The model under review builds one solid part; all positions refer to its coordinate system, in mm. A direction names the side the tool comes from. Round coordinates to 2 decimals unless told otherwise and drop trailing zeros. Write each loop counter-clockwise with the first axis right and the second up, starting at its lowest first coordinate (ties: lowest second). Pieces come first, ordered by that corner, then holes.
Item 1: Add section A-A (y = 7). Give the boundary of the cut face in (x, z), plus the area to 3 significant figures.
Item 2: Machinability: for faces 4 (the face through (2, 6, -27)), 5 (the face through (-5.93, 11.055, -13.579)), 6 (the face through (-0.493, 11.562, -13.026)), which of the approach directions +Z, -Z, +X, -X, +Y, -Y give a long, thin tool a straight path to every point of the face, cutting with its end or side? Answer none if there is none.
Item 3: Add section B-B (z = 0). Give the boundary of the cut face in (x, y).
Item 4: Clearance check with flat-ended pins moving along their axes: pin 1 Ø5 at (y, z) = (10, 0) entering from -X; pin 2 Ø3 at (x, y) = (-8.5, 6.5) entering from +Z; pin 3 Ø1.5 at (x, y) = (-6, 4) entering from +Z. State where each tip first meets the part, or that it passes through.
Item 5: Add section C-C (y = 10). Give the boundary of the cut face in (x, z).
Item 6: Add section D-D (x = -3). Give the boundary of the cut face in (y, z).
Item 7: To check wall thickness, follow L1, parallel to Y at x = 1.3, z = 0; L2, parallel to Z at x = 3.05, y = 10; L3, parallel to X at y = 10.5, z = -23. State the ranges of each line that lie inside material, in increasing order.
Item 8: Draft analysis for pull direction Z (two halves, no side actions). For faces 1 (the face through (2, 16, -12)), 2 (the face through (2, 2, 0)), 3 (the face through (2, 6, 3)), state which applies: +Z half, -Z half, draft (parallel to the pull), parting line (faces both ways), or undercut.
Autodesk Fusion 360 part; units mm, degrees
sketch "Sketch1" plane through (0, 0, 0) normal (1, 0, 0) x (0, 0, -1)
  circle A0 centre (0, 0) radius 2
  line L0 (0.0008, 2) -> (0.0008, 8)
  line L1 (0.0008, 8) -> (0.0008, 10)
  circle A1 centre (0.0008, 10) radius 2
  line L2 (-3, 15) -> (27, 15)
  line L3 (27, 15) -> (27, -3)
  line L4 (27, -3) -> (-3, -3)
  line L5 (-3, -3) -> (-3, 15)
  circle A2 centre (18.0008, 7) radius 6
  circle A3 centre (18.0008, 7) radius 6.75
  dimension "d1" = 4
  dimension "d2" = 6
  dimension "d3" = 2
  dimension "d4" = 4
  dimension "d6" = 30
  dimension "d7" = 18
  dimension "d33" = 12
  dimension "d34" = 13.5
  dimension "d42" = 10
  dimension "d43" = 3
extrude "Extrude1" add sketch "Sketch1" along normal blind 4 contours L2 L3 L4 L5 | A2 | A3
extrude "Extrude2" add 1 faces at (1.3333, 15, -7) along direction (0, 1, 0) blind 1
extrude "Extrude3" add 1 faces at (1.3333, -3, -17) along direction (0, -1, 0) blind 1
extrude "Extrude8" add sketch "Sketch1" against normal blind 12 contours A2
extrude "Extrude9" add sketch "Sketch1" against normal blind 1 contours A3
sketch "Sketch5" plane through (-12, 0, 0) normal (-1, 0, 0) x (0, 0, 1)
  circle A0 centre (-18.0008, 7) radius 6
  circle A1 centre (-18.0008, 7) radius 6.75
  dimension "d39" = 13.5
extrude "Extrude10" add sketch "Sketch5" against normal blind 1
Numbers:
1. outline: (-12, -24.75) - (-11, -24.75) - (-11, -24) - (-1, -24) - (-1, -24.75) - (0, -24.75) - (0, -27) - (4, -27) - (4, 3) - (0, 3) - (0, -11.25) - (-1, -11.25) - (-1, -12) - (-11, -12) - (-11, -11.25) - (-12, -11.25) - close
1. area: 267 mm2
2. face 4: -Z, +X, -X, +Y, -Y
2. face 5: none
2. face 6: -X
3. outline: (0, -4) - (4, -4) - (4, -2) - (0, -2) - close; (0, 2) - (4, 2) - (4, 8) - (0, 8) - close; (0, 12) - (4, 12) - (4, 16) - (0, 16) - close
4. pin 1: stops at x = 0
4. pin 2: stops at z = -12
4. pin 3: stops at z = -12.44
5. outline: (-12, -24.05) - (-11, -24.05) - (-11, -23.2) - (-1, -23.2) - (-1, -24.05) - (0, -24.05) - (0, -27) - (4, -27) - (4, -2) - (0, -2) - (0, -11.95) - (-1, -11.95) - (-1, -12.8) - (-11, -12.8) - (-11, -11.95) - (-12, -11.95) - close; (0, 2) - (4, 2) - (4, 3) - (0, 3) - close
6. outline: circle Ø12 at (7, -18)
7. L1: y = -4 to -2, 2 to 8, 12 to 16
7. L2: z = -27 to -2, 2 to 3
7. L3: x = -12 to -11, -1 to 4
8. face 1: draft
8. face 2: undercut
8. face 3: +Z half
